Model file for the job. Use its own axes, mm. A direction names the side the tool comes from. Coordinates: 2 decimals unless noted, no trailing zeros. Order: outer loops, then holes, each group sorted by start corner. A loop starts at its lowest first (then second) coordinate and runs counter-clockwise, first axis right, second up. Notation, with made-up numbers: (-26.75, -34.75) -> (1.25, -34.75) arc R6 cw to (1.25, -25.75) -> close; hole circle Ø7 at (17.25, 51.25). An arc over 180 degrees is marked (long way). Write item = value, one per line. Start each with the question number.
Q1. Flat gauge pins, fed straight in: pin 1 (5.5 mm diameter, centred on x = -59, y = 9.5, fed in from +Z); pin 2 (6 mm diameter, centred on x = -174.5, y = 9.5, fed in from -Z); pin 3 (6.5 mm diameter, centred on x = -140, y = 10, fed in from +Z); pin 4 (11 mm diameter, centred on x = -180, y = 10, fed in from -Z). Where does each tip first touch, or does it go through?
Q2. Wall check: line 1 (Y direction, x = -20, z = 117.5); line 2 (Z direction, x = -115, y = 2); line 3 (X direction, y = 14.75, z = 15). Give the ranges that are in metal, low to high. Write a range as from..to.
Q3. 3-axis set-ups, long thin cutter, end or side, ignore diameter. For faces 1 (the face through (-40, 10, 30)), 2 (the face through (-143.34, 11.05, 119.72)), 3 (the face through (-37.71, 0.79, 2.35)): which of +Z, -Z, +X, -X, +Y, -Y reach the whole face in a straight line?
Q4. Cut at B-B, the plane x = -140. List the corners of the cut face in (y, z), plus the area to 3 significant figures.
Q5. Cut at A-A, the plane z = 40. List the corners of the cut face in (x, y), plus the area to 3 significant figures.
Q6. Mould opens along X. For faces 4 (the face through (-179.241, 6.583, 119.72)), 5 (the face through (-20, 10, 0)), 6 (the face through (-190.244, 19.681, 75.197)) say: +X half, -X half, draft (parallel to the pull), parting line (faces both ways), or undercut.
Q7. Cut at D-D, the plane z = 128.5. List the corners of the cut face in (x, y).
Q8. Cut at C-C, the plane y = 10. List the corners of the cut face in (x, z), plus the area to 3 significant figures.
from build123d import *

# Parameters (mm, degrees)
BOSS_EXTRUDE1_DEPTH      = 20
FILLET1_R                = 10
M6_CLEARANCE_HOLE1_D     = 7
M6_CLEARANCE_HOLE1_DEPTH = 40
FILLET2_R                = 5
FILLET3_R                = 30
CHAMFER1_SIZE            = 2


with BuildPart() as part:
    # Sketch1 → Boss-Extrude1 (new body)
    with BuildSketch(Plane(origin=(0, 0, 0), x_dir=(1, 0, 0), z_dir=(0, 1, 0))):
        Polygon((0, 0), (0, -140), (-200, -140), (-200, -65), (-40, -65), (-40, 0), align=None)
    extrude(amount=BOSS_EXTRUDE1_DEPTH)

    # Fillet1
    fillet1_edges = [part.edges().sort_by_distance(p)[0] for p in [
        (-40, 10, 65),
    ]]
    fillet(fillet1_edges, radius=FILLET1_R)

    # M6 Clearance Hole1
    with Locations(Plane(origin=(10895.274804619, -492.997703293, 140), x_dir=(1, 0, 0), z_dir=(0, 0, 1))):
        with Locations((-11075.274804618, 502.997703293), (-11035.274804618, 502.997703293), (-10955.274804618, 502.997703293), (-10915.274804618, 502.997703293)):
            Hole(M6_CLEARANCE_HOLE1_D / 2, depth=M6_CLEARANCE_HOLE1_DEPTH)

    # Fillet2
    fillet2_edges = [part.edges().sort_by_distance(p)[0] for p in [
        (0, 10, 0),
        (-40, 10, 0),
    ]]
    fillet(fillet2_edges, radius=FILLET2_R)

    # Fillet3
    fillet3_edges = [part.edges().sort_by_distance(p)[0] for p in [
        (-200, 10, 65),
    ]]
    fillet(fillet3_edges, radius=FILLET3_R)

    # Chamfer1
    chamfer1_edges = [part.edges().sort_by_distance(p)[0] for p in [
        (-110, 0, 65),
        (-110, 20, 65),
        (-100, 20, 140),
        (-42.928932188, 0, 62.071067812),
        (-42.928932188, 20, 62.071067812),
        (0, 20, 72.5),
        (-20, 0, 0),
        (-20, 20, 0),
        (-40, 0, 30),
        (-38.535533906, 0, 1.464466094),
        (-1.464466094, 0, 1.464466094),
        (-40, 20, 30),
        (-38.535533906, 20, 1.464466094),
        (-1.464466094, 20, 1.464466094),
        (-200, 0, 117.5),
        (-200, 20, 117.5),
        (-191.213203436, 0, 73.786796564),
        (-191.213203436, 20, 73.786796564),
        (0, 0, 72.5),
        (-100, 0, 140),
    ]]
    chamfer(chamfer1_edges, length=CHAMFER1_SIZE)


solid = part.part
Here are the results:
q1.pin_1 = 140
q1.pin_2 = 65.04
q1.pin_3 = 100
q1.pin_4 = 65.34
q2.line_1 = 0..6.5, 13.5..20
q2.line_2 = 65..140
q2.line_3 = -40..0
q3.face_1 = -Z, -X, +Y, -Y
q3.face_2 = +Z
q3.face_3 = -Z, -X, -Y
q4.outline = (0, 67) -> (2, 65) -> (18, 65) -> (20, 67) -> (20, 138) -> (18, 140) -> (13.5, 140) -> (13.5, 100) -> (6.5, 100) -> (6.5, 140) -> (2, 140) -> (0, 138) -> close
q4.area = 1,210 mm²
q5.outline = (-40, 2) -> (-38, 0) -> (-2, 0) -> (0, 2) -> (0, 18) -> (-2, 20) -> (-38, 20) -> (-40, 18) -> close
q5.area = 792 mm²
q6.face_4 = undercut
q6.face_5 = draft
q6.face_6 = -X half
q7.outline = (-200, 2) -> (-198, 0) -> (-2, 0) -> (0, 2) -> (0, 18) -> (-2, 20) -> (-198, 20) -> (-200, 18) -> close; hole circle Ø7 at (-180, 10); hole circle Ø7 at (-140, 10); hole circle Ø7 at (-60, 10); hole circle Ø7 at (-20, 10)
q8.outline = (-200, 95) arc R30 ccw to (-170, 65) -> (-50, 65) arc R10 cw to (-40, 55) -> (-40, 5) arc R5 ccw to (-35, 0) -> (-5, 0) arc R5 ccw to (0, 5) -> (0, 140) -> (-16.5, 140) -> (-16.5, 100) -> (-23.5, 100) -> (-23.5, 140) -> (-56.5, 140) -> (-56.5, 100) -> (-63.5, 100) -> (-63.5, 140) -> (-136.5, 140) -> (-136.5, 100) -> (-143.5, 100) -> (-143.5, 140) -> (-176.5, 140) -> (-176.5, 100) -> (-183.5, 100) -> (-183.5, 140) -> (-200, 140) -> close
q8.area = 16,300 mm²
